Input: part model. Units: mm. Frame: model coordinates. Face numbers are marked on the shaded views. A direction names the side the tool comes from. Give positions to 0.01 mm unless a question says otherwise; leave off trailing zeros. Loops run counter-clockwise (first coordinate to the right, second up) from the corner with the lowest first, then second, coordinate; pieces in that order, holes last. Notation, with made-up numbers: M 10,-23.5 L 52,-23.5 A24 cw 52,-12.5 Z; hole C 3.5,-15.5 d9. An arc over 180 degrees is marked long. One line per item, written item: value. Start each with the question number.
(1) Section C-C on z = -51.5. Output: boundary loops of the cut face in (x, y).
(2) Pin query (flat end, axial travel): P1, Ø12, axis at x = -5.5, z = -65, coming from the -Y side; P2, Ø3, axis at x = 3.5, y = -1.5, coming from the +Z side; P3, Ø8, axis at x = 8, y = 7, coming from the +Z side; P4, Ø1.5, axis at y = 3.5, z = -48.5, coming from the +X side. Return the tip coordinate at first contact, or that it passes through.
(3) Section A-A on z = -75. Output: boundary loops of the cut face in (x, y).
(4) Ray query, line 1 along X through (y, z) = (-15, -65.5); line 2 along Z through (x, y) = (-9, 35); line 3 along Y through (x, z) = (4, -54). Return the intervals inside material, ascending. Write a range as from..to.
(5) Section D-D on y = 23. Output: boundary loops of the cut face in (x, z).
(6) Pull-direction query (X, two-part tool) for the marked faces 1, 2, 3 and 4; classes: released by +X, released by -X, zero draft, split by the parting line, or undercut.
(7) Access query for the marked faces 5, 6 and 7. Directions: +Z, -Z, +X, -X, +Y, -Y. A direction counts if a zero-diameter tool reaches every point of the face in a straight line with its end or side. Return the directions, or none.
(8) Section B-B on y = 15. Output: boundary loops of the cut face in (x, z), plus the area to 3 significant figures.
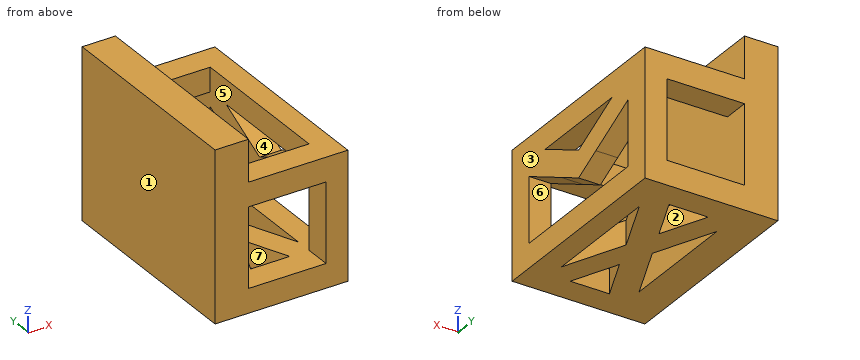
```python
from build123d import *

# Parameters (mm, degrees)
BOSS_EXTRUDE2_DEPTH      = 0.25
BOSS_EXTRUDE2_DEPTH_BACK = 38
SKETCH1_W                = 8.8
SKETCH1_H                = 54.5
BOSS_EXTRUDE3_DEPTH      = 6.35
SKETCH3_W                = 5.75
SKETCH3_H                = 54.5
BOSS_EXTRUDE4_DEPTH      = 6.35
BOSS_EXTRUDE5_DEPTH      = 5.75


with BuildPart() as part:
    # Sketch1 → Boss-Extrude2 (new, two sides: drawn at the far end of the back side and taken through both)
    with BuildSketch(Plane(origin=(0, 0, -77.8375), x_dir=(-1, 0, 0), z_dir=(0, 0, -1)).offset(-BOSS_EXTRUDE2_DEPTH_BACK)):
        with Locations((14.65, 10)):
            Rectangle(SKETCH1_W, SKETCH1_H)
    extrude(amount=BOSS_EXTRUDE2_DEPTH + BOSS_EXTRUDE2_DEPTH_BACK)

    # Sketch2 → Boss-Extrude3 (add)
    with BuildSketch(Plane(origin=(0, 0, -50.8375), x_dir=(-1, 0, 0), z_dir=(0, 0, -1))):
        Polygon((10.25, -17.25), (10.25, -10.25), (-10.25, -10.25), (-10.25, 30.25), (10.25, 30.25), (10.25, 37.25), (-16, 37.25), (-16, -17.25), align=None)
    extrude(amount=BOSS_EXTRUDE3_DEPTH)

    # Sketch3 → Boss-Extrude4 (add)
    with BuildSketch(Plane(origin=(0, 0, -78.0875), x_dir=(-1, 0, 0), z_dir=(0, 0, -1))):
        Polygon((10.25, 30.25), (10.25, 37.25), (-10.25, 37.25), (-10.25, 30.25), (-5.17, 30.25), (5.17, 30.25), align=None)
        with Locations((-13.125, 10)):
            Rectangle(SKETCH3_W, SKETCH3_H)
        Polygon((19.05, -17.25), (19.05, 37.25), (10.25, 37.25), (10.25, 30.25), (10.25, 25.971389376), (10.25, -5.971389376), (10.25, -10.25), (10.25, -17.25), align=None)
        Polygon((10.25, 25.971389376), (10.25, 30.25), (5.17, 30.25), (0, 18.105733912), (3.450735024, 10), align=None)
        Polygon((-5.17, 30.25), (-10.25, 30.25), (-10.25, 25.971389376), (-3.450735024, 10), (0, 18.105733912), align=None)
        Polygon((0, 1.894266088), (3.450735024, 10), (0, 18.105733912), (-3.450735024, 10), align=None)
        Polygon((-10.25, -5.971389376), (-10.25, -10.25), (-5.17, -10.25), (0, 1.894266088), (-3.450735024, 10), align=None)
        Polygon((5.17, -10.25), (10.25, -10.25), (10.25, -5.971389376), (3.450735024, 10), (0, 1.894266088), align=None)
        Polygon((-10.25, -17.25), (10.25, -17.25), (10.25, -10.25), (5.17, -10.25), (-5.17, -10.25), (-10.25, -10.25), align=None)
    extrude(amount=BOSS_EXTRUDE4_DEPTH)

    # Sketch4 → Boss-Extrude5 (add)
    with BuildSketch(Plane(origin=(16, 0, 0), x_dir=(0, 0, -1), z_dir=(1, 0, 0))):
        Polygon((67.6375, 2.939263745), (64.082844513, 10), (57.1875, -3.696463464), (57.1875, -10.25), (60.9975, -10.25), align=None)
        Polygon((60.9975, -10.25), (57.1875, -10.25), (57.1875, -17.25), (78.0875, -17.25), (78.0875, -10.25), (74.2775, -10.25), align=None)
        Polygon((71.192155487, 10), (67.6375, 17.060736255), (64.082844513, 10), (67.6375, 2.939263745), align=None)
        Polygon((78.0875, 37.25), (57.1875, 37.25), (57.1875, 30.25), (60.9975, 30.25), (74.2775, 30.25), (78.0875, 30.25), align=None)
        Polygon((60.9975, 30.25), (57.1875, 30.25), (57.1875, 23.696463464), (64.082844513, 10), (67.6375, 17.060736255), align=None)
    extrude(amount=-BOSS_EXTRUDE5_DEPTH)


solid = part.part
```
Output values:
1. outline: M -19.05,-17.25 L 16,-17.25 L 16,37.25 L -19.05,37.25 Z; hole M -10.25,-10.25 L 10.25,-10.25 L 10.25,30.25 L -10.25,30.25 Z
2. P1: stops at y = -17.25
2. P2: stops at z = -78.09
2. P3: stops at z = -50.84
2. P4: stops at x = -10.25
3. outline: M -19.05,-17.25 L -10.25,-17.25 L -10.25,37.25 L -19.05,37.25 Z; M 10.25,-17.25 L 16,-17.25 L 16,-10.25 L 10.25,-10.25 Z; M 10.25,30.25 L 16,30.25 L 16,37.25 L 10.25,37.25 Z
4. line 1: x = -19.05..-10.25, 10.25..16
4. line 2: z = -84.44..-78.09, -57.19..-50.84
4. line 3: y = -17.25..-10.25, 30.25..37.25
5. outline: M -19.05,-84.44 L -10.25,-84.44 L -10.25,-39.84 L -19.05,-39.84 Z; M -8.99,-84.44 L -2.08,-84.44 L -2.08,-78.09 L -8.99,-78.09 Z; M 2.08,-84.44 L 8.99,-84.44 L 8.99,-78.09 L 2.08,-78.09 Z; M 10.25,-84.44 L 16,-84.44 L 16,-78.09 L 10.25,-78.09 Z; M 10.25,-64.65 L 16,-64.65 L 16,-57.54 L 10.25,-57.54 Z; M 10.25,-57.19 L 16,-57.19 L 16,-50.84 L 10.25,-50.84 Z
6. face 1: released by -X
6. face 2: undercut
6. face 3: released by +X
6. face 4: zero draft
7. face 5: none
7. face 6: +X
7. face 7: +Z, -Z
8. outline: M -19.05,-84.44 L -10.25,-84.44 L -10.25,-39.84 L -19.05,-39.84 Z; M -5.58,-84.44 L 5.58,-84.44 L 5.58,-78.09 L -5.58,-78.09 Z; M 10.25,-84.44 L 16,-84.44 L 16,-78.09 L 10.25,-78.09 Z; M 10.25,-68.67 L 16,-68.67 L 16,-61.57 L 10.25,-61.57 Z; M 10.25,-57.19 L 16,-57.19 L 16,-50.84 L 10.25,-50.84 Z
8. area: 577 mm²
